from build123d import *

# Parameters (mm, degrees)
SKETCH_1_W                  = 74
SKETCH_1_H                  = 74
EXTRUDE_1_DEPTH             = 10
SKETCH_2_W                  = 71
SKETCH_2_H                  = 71
CUT_EXTRUDE_1_DEPTH         = 8.5
SKETCH_3_R                  = 3.5
EXTRUDE_2_DEPTH             = 7
SKETCH_4_R                  = 1.25
CUT_EXTRUDE_2_DEPTH         = 7
SKETCH_5_W                  = 5
SKETCH_5_H                  = 2
EXTRUDE_3_DEPTH             = 0.5
CHAMFER_1_SIZE              = 0.5
CHAMFER_1_SIZE2             = 1.37373871
CHAMFER_1_OF_MIRROR_1_SIZE2 = 1.37373871
CHAMFER_1_OF_MIRROR_1_SIZE  = 0.5
SKETCH_6_W                  = 15
SKETCH_6_H                  = 6
EXTRUDE_4_DEPTH             = 60
FILLET_1_R                  = 10
SKETCH_8_R                  = 15
EXTRUDE_5_DEPTH             = 20
EXTRUDE_5_DIRECTION_2_REACH = 106.169
SKETCH_9_W                  = 15
SKETCH_9_H                  = 30
CUT_EXTRUDE_3_DEPTH         = 121.939034228
SKETCH_10_R                 = 11
CUT_EXTRUDE_4_DEPTH         = 108.197248099
FILLET_2_R                  = 50
CUT_EXTRUDE_5_DEPTH         = 155.477344617
CUT_EXTRUDE_5_DEPTH_BACK    = 155.477344617
SKETCH_11_R                 = 2.5
SWEEP_START                 = -53
SWEEP_1_DEPTH               = 17.335664095
SKETCH_18_R                 = 0.5
CUT_EXTRUDE_7_DEPTH         = 107.843343379


with BuildPart() as part:
    # Эскиз1 → Бобышка-Вытянуть1 (new body)
    with BuildSketch(Plane(origin=(0, 0, 0), x_dir=(1, 0, 0), z_dir=(0, 1, 0))):
        Rectangle(SKETCH_1_W, SKETCH_1_H)
    extrude(amount=-EXTRUDE_1_DEPTH)

    # Эскиз2 → Вырез-Вытянуть1 (cut)
    with BuildSketch(Plane(origin=(0, 0, 0), x_dir=(1, 0, 0), z_dir=(0, 1, 0))):
        Rectangle(SKETCH_2_W, SKETCH_2_H)
    extrude(amount=-CUT_EXTRUDE_1_DEPTH, mode=Mode.SUBTRACT)

    # Эскиз3 → Бобышка-Вытянуть2 (add)
    with BuildSketch(Plane(origin=(0, -8.5, 0), x_dir=(1, 0, 0), z_dir=(0, 1, 0))):
        with Locations(Location((-30, 30, 0), (0, 0, 270))):
            Circle(SKETCH_3_R)
        with Locations(Location((30, 30, 0), (0, 0, 90))):
            Circle(SKETCH_3_R)
        with Locations(Location((30, -30, 0), (0, 0, 270))):
            Circle(SKETCH_3_R)
        with Locations(Location((-30, -30, 0), (0, 0, 90))):
            Circle(SKETCH_3_R)
    extrude(amount=EXTRUDE_2_DEPTH)

    # Эскиз4 → Вырез-Вытянуть2 (cut)
    with BuildSketch(Plane(origin=(0, -1.5, 0), x_dir=(1, 0, 0), z_dir=(0, 1, 0))):
        with Locations(Location((-30, 30, 0), (0, 0, 270))):
            Circle(SKETCH_4_R)
        with Locations(Location((-30, -30, 0), (0, 0, 270))):
            Circle(SKETCH_4_R)
        with Locations(Location((30, 30, 0), (0, 0, 270))):
            Circle(SKETCH_4_R)
        with Locations(Location((30, -30, 0), (0, 0, 270))):
            Circle(SKETCH_4_R)
    extrude(amount=-CUT_EXTRUDE_2_DEPTH, mode=Mode.SUBTRACT)

    # Эскиз5 → Бобышка-Вытянуть3 (add)
    with BuildSketch(Plane.XY.offset(37)):
        with Locations((0, -1)):
            Rectangle(SKETCH_5_W, SKETCH_5_H)
    extrude_3 = extrude(amount=EXTRUDE_3_DEPTH)

    # Фаска1
    chamfer_1_edges = [part.edges().sort_by_distance(p)[0] for p in [
        (0, 0, 37.5),
    ]]
    chamfer_1_side = [part.faces().sort_by_distance(p)[0] for p in [
        (0, 0, -35.949940478),
    ]]
    chamfer(chamfer_1_edges, length=CHAMFER_1_SIZE, length2=CHAMFER_1_SIZE2, reference=chamfer_1_side[0])

    # Зеркальное отражение1: Бобышка-Вытянуть3 across plane
    add(extrude_3.mirror(Plane.XY))

    # Фаска1 of Зеркальное отражение1
    chamfer_1_of_mirror_1_edges = [part.edges().sort_by_distance(p)[0] for p in [
        (0, 0, -37.5),
    ]]
    chamfer(chamfer_1_of_mirror_1_edges, length=CHAMFER_1_OF_MIRROR_1_SIZE, length2=CHAMFER_1_OF_MIRROR_1_SIZE2)

    # Эскиз6 → Бобышка-Вытянуть4 (add)
    with BuildSketch(Plane.ZY.offset(37)):
        with Locations((0, -7)):
            Rectangle(SKETCH_6_W, SKETCH_6_H)
    extrude(amount=EXTRUDE_4_DEPTH)

    # Скругление1
    fillet_1_edges = [part.edges().sort_by_distance(p)[0] for p in [
        (-37, -7, 7.5),
        (-37, -7, -7.5),
    ]]
    fillet(fillet_1_edges, radius=FILLET_1_R)

    # Эскиз8 → Бобышка-Вытянуть5 (add)
    with BuildSketch(Plane(origin=(0, -4, 0), x_dir=(0, 0, -1), z_dir=(0, 1, 0))):
        with Locations(Location((0, 97, 0), (0, 0, 180))):
            Circle(SKETCH_8_R)
    extrude(amount=EXTRUDE_5_DEPTH)

    # Бобышка-Вытянуть5 direction 2: up to this face of the body (flat: up to its plane)
    extrude_5_direction_2_end = Plane(part.part.faces().sort_by_distance((-9.656440707, -10, 0))[0])
    # Эскиз8 → Бобышка-Вытянуть5 direction 2 (add, up to the picked face)
    with BuildSketch(Plane(origin=(0, -4, 0), x_dir=(0, 0, -1), z_dir=(0, 1, 0)), mode=Mode.PRIVATE) as extrude_5_direction_2_sk1:
        with Locations(Location((0, 97, 0), (0, 0, 180))):
            Circle(SKETCH_8_R)
    extrude_5_direction_2_tool1 = split(extrude(extrude_5_direction_2_sk1.sketch, amount=-EXTRUDE_5_DIRECTION_2_REACH, mode=Mode.PRIVATE), bisect_by=extrude_5_direction_2_end, keep=Keep.BOTH, mode=Mode.PRIVATE)
    add(extrude_5_direction_2_tool1.solids().sort_by(Axis((-97, -4, 0), (0, -1, 0)))[0])

    # Эскиз9 → Вырез-Вытянуть3 (cut, through all)
    with BuildSketch(Plane(origin=(0, 16, 0), x_dir=(1, 0, 0), z_dir=(0, 1, 0))):
        with Locations((-104.5, 0)):
            Rectangle(SKETCH_9_W, SKETCH_9_H)
    extrude(amount=-CUT_EXTRUDE_3_DEPTH, mode=Mode.SUBTRACT)

    # Эскиз10 → Вырез-Вытянуть4 (cut, through all)
    with BuildSketch(Plane(origin=(0, 16, 0), x_dir=(1, 0, 0), z_dir=(0, 1, 0))):
        with Locations((-97, 0)):
            Circle(SKETCH_10_R)
    extrude(amount=-CUT_EXTRUDE_4_DEPTH, mode=Mode.SUBTRACT)

    # Скругление2
    fillet_2_edges = [part.edges().sort_by_distance(p)[0] for p in [
        (-84.009618943, -7, -7.5),
        (-84.009618943, -7, 7.5),
    ]]
    fillet(fillet_2_edges, radius=FILLET_2_R)

    # Эскиз11 → Вырез-Вытянуть5 (cut, two sides: drawn at the far end of the back side and taken through both)
    with BuildSketch(Plane(origin=(-112, 0, 0), x_dir=(0, 0, 1), z_dir=(1, 0, 0)).offset(-CUT_EXTRUDE_5_DEPTH_BACK)):
        with Locations((0, -8.5)):
            Circle(SKETCH_11_R)
    extrude(amount=CUT_EXTRUDE_5_DEPTH + CUT_EXTRUDE_5_DEPTH_BACK, mode=Mode.SUBTRACT)

    # Вырез-По траектории1: read off the stored shape, not the designer's step
    # Вырез-По траектории1 outline → Вырез-По траектории1 (cut)
    with BuildSketch(Plane(origin=(0, 0, 0), x_dir=(-0.27037806600999104, 0.962753255180235, -0.0013678671566966505), z_dir=(0.9627409348714416, 0.27038152606985083, 0.004870593701078593)).offset(SWEEP_START)):
        with BuildLine():
            add(Edge.make_bspline(
                [(2.861200358, -1.320385383), (5.749460123, -1.320385383), (5.745356522, 1.679576226), (2.857096756, 1.679576226), (-0.031163009, 1.679576226), (-0.027059408, -1.320385383), (2.861200358, -1.320385383)],
                knots=[0, 0, 0, 0, 0.5, 0.5, 0.5, 1, 1, 1, 1], degree=3, weights=[1, 0.333333333, 0.333333333, 1, 0.333333333, 0.333333333, 1]))
        make_face()
    extrude(amount=SWEEP_1_DEPTH, mode=Mode.SUBTRACT)

    # Эскиз18 → Вырез-Вытянуть7 (cut, through all)
    with BuildSketch(Plane(origin=(0, -8.5, 0), x_dir=(1, 0, 0), z_dir=(0, 1, 0))):
        with Locations(Location((-35, 35, 0), (0, 0, 270))):
            Circle(SKETCH_18_R)
        with Locations(Location((-21, 35, 0), (0, 0, 270))):
            Circle(SKETCH_18_R)
        with Locations(Location((-7, 35, 0), (0, 0, 270))):
            Circle(SKETCH_18_R)
        with Locations(Location((7, 35, 0), (0, 0, 270))):
            Circle(SKETCH_18_R)
        with Locations(Location((21, 35, 0), (0, 0, 270))):
            Circle(SKETCH_18_R)
        with Locations(Location((35, 35, 0), (0, 0, 270))):
            Circle(SKETCH_18_R)
        with Locations(Location((-21, 11.666666667, 0), (0, 0, 270))):
            Circle(SKETCH_18_R)
        with Locations(Location((-7, 11.666666667, 0), (0, 0, 270))):
            Circle(SKETCH_18_R)
        with Locations(Location((7, 11.666666667, 0), (0, 0, 270))):
            Circle(SKETCH_18_R)
        with Locations(Location((21, 11.666666667, 0), (0, 0, 270))):
            Circle(SKETCH_18_R)
        with Locations(Location((35, 11.666666667, 0), (0, 0, 270))):
            Circle(SKETCH_18_R)
        with Locations(Location((-21, -11.666666667, 0), (0, 0, 270))):
            Circle(SKETCH_18_R)
        with Locations(Location((-7, -11.666666667, 0), (0, 0, 270))):
            Circle(SKETCH_18_R)
        with Locations(Location((7, -11.666666667, 0), (0, 0, 270))):
            Circle(SKETCH_18_R)
        with Locations(Location((21, -11.666666667, 0), (0, 0, 270))):
            Circle(SKETCH_18_R)
        with Locations(Location((35, -11.666666667, 0), (0, 0, 270))):
            Circle(SKETCH_18_R)
        with Locations(Location((-21, -35, 0), (0, 0, 270))):
            Circle(SKETCH_18_R)
        with Locations(Location((-7, -35, 0), (0, 0, 270))):
            Circle(SKETCH_18_R)
        with Locations(Location((7, -35, 0), (0, 0, 270))):
            Circle(SKETCH_18_R)
        with Locations(Location((21, -35, 0), (0, 0, 270))):
            Circle(SKETCH_18_R)
        with Locations(Location((35, -35, 0), (0, 0, 270))):
            Circle(SKETCH_18_R)
        with Locations(Location((-35, 11.666666667, 0), (0, 0, 270))):
            Circle(SKETCH_18_R)
        with Locations(Location((-35, -11.666666667, 0), (0, 0, 270))):
            Circle(SKETCH_18_R)
        with Locations(Location((-35, -35, 0), (0, 0, 270))):
            Circle(SKETCH_18_R)
    extrude(amount=-CUT_EXTRUDE_7_DEPTH, mode=Mode.SUBTRACT)


solid = part.part
Could you check a few things on this model? Use its own coordinates, in mm. A direction names the side the tool comes from. Give positions to 0.01 mm unless a question says otherwise; leave off trailing zeros. Loops run counter-clockwise (first coordinate to the right, second up) from the corner with the lowest first, then second, coordinate; pieces in that order, holes last. Notation, with made-up numbers: (-4, -12.75) -> (41, -12.75) arc R25 ccw to (41, 22.25) -> close; hole circle Ø10 at (-25.5, 46). An arc over 180 degrees is marked (long way). Answer as CSV lines item,"result". Start each with the question number.
(1) Which directions (+Z, -Z, +X, -X, +Y, -Y) give clear straight access to the entire face, cutting with the end or side of a thin tool? Please do faces 5 (the flat face through (-17, 0, -36)), 6 (the flat face through (37, -5, 1)), 7 (the flat face through (30, -8.5, 30)), 8 (the flat face through (-57, -7, 7.5)).
(2) We'd pull the mould along Z, two halves only. Please class faces 1 (the cylindrical face through (-39.85, -6.96, -10.51)), 2 (the cylindrical face through (-78.863, -6.958, 9.005)), 3 (the flat face through (-28, -1.5, 30)), 4 (the flat face through (-97, 3, -13)): released by +Z, released by -Z, zero draft, split by the parting line, or undercut.
(3) If we section it at A-A on x = -13: Write out the boundary of the cut face in (y, z), then the cut area to 4 significant figures.
(4) I'm going to push flat-ended pins straight in: pin 1 Ø8 at (x, z) = (12.5, -14) entering from +Y; pin 2 Ø12 at (x, y) = (-46, -7) entering from +Z; pin 3 Ø1.8 at (x, y) = (-57.5, -8) entering from +Z. Where does each tip first touch, or does it pass through?
(5) I need wall thicknesses on probe 1 along Z at (x, y) = (35, -9.65); probe 2 along X at (y, z) = (-0.5, 34); probe 3 along X at (y, z) = (-2, 12.5). Which ranges of each line are inside material? Lowest first, please.
(6) If we section it at D-D on x = 30: Write out the boundary of the cut face in (y, z), then the cut area to 4 significant figures.
(7) If we section it at C-C on z = 24: Write out the boundary of the cut face in (x, y).
(8) If we section it at B-B on y = 8.5: Write out the boundary of the cut face in (x, z), then the cut area to 3 significant figures.
Computed:
1,face 5,"+Z, -Z, +X, +Y"
1,face 6,"+Z, -Z, +X, +Y, -Y"
1,face 7,"+Y"
1,face 8,"+Z, +Y, -Y"
2,face 1,"released by -Z"
2,face 2,"released by +Z"
2,face 3,"undercut"
2,face 4,"zero draft"
3,outline,"(-10, -37) -> (0, -37) -> (0, -35.5) -> (-8.5, -35.5) -> (-8.5, 35.5) -> (0, 35.5) -> (0, 37) -> (-10, 37) -> close"
3,area,"136.5 mm2"
4,pin 1,"stops at y = -8.5"
4,pin 2,"stops at z = 10.36"
4,pin 3,"stops at z = 7.5"
5,probe 1,"z = -37 to -35.5, -34.5 to -12.17, -11.17 to 11.17, 12.17 to 34.5, 35.5 to 37"
5,probe 2,"x = -37 to -35.5, 35.5 to 37"
5,probe 3,"x = -97 to -88.71, -37 to -35.5, 35.5 to 37"
6,outline,"(-10, -37) -> (0, -37) -> (0, -35.5) -> (-8.5, -35.5) -> (-8.5, -33.5) -> (-1.5, -33.5) -> (-1.5, -31.25) -> (-8.5, -31.25) -> (-8.5, -28.75) -> (-1.5, -28.75) -> (-1.5, -26.5) -> (-8.5, -26.5) -> (-8.5, 26.5) -> (-1.5, 26.5) -> (-1.5, 28.75) -> (-8.5, 28.75) -> (-8.5, 31.25) -> (-1.5, 31.25) -> (-1.5, 33.5) -> (-8.5, 33.5) -> (-8.5, 35.5) -> (0, 35.5) -> (0, 37) -> (-10, 37) -> close"
6,area,"199.5 mm2"
7,outline,"(-37, -10) -> (37, -10) -> (37, 0) -> (35.5, 0) -> (35.5, -8.5) -> (-35.5, -8.5) -> (-35.5, 0) -> (-37, 0) -> close"
8,outline,"(-97, -15) arc R15 ccw to (-82.21, -2.5) -> (-86.29, -2.5) arc R11 cw to (-97, -11) -> close; (-97, 11) arc R11 cw to (-86.29, 2.5) -> (-82.21, 2.5) arc R15 ccw to (-97, 15) -> close"
8,area,"143 mm2"
